Geometry: final body of the model. Coordinates: model frame, mm. A direction names the side the tool comes from. Coordinates: 2 decimals unless noted, no trailing zeros. Order: outer loops, then holes, each group sorted by start corner. A loop starts at its lowest first (then second) coordinate and runs counter-clockwise, first axis right, second up. Notation, with made-up numbers: (-27.75, -34.75) -> (4.25, -34.75) arc R11 ccw to (4.25, -17.75) -> close; hole circle Ø8 at (55.25, -1.75). An arc over 180 degrees is marked (long way). Answer in a Markdown table with one row per item. Add a question column.
1) Section query B-B on y = -0.5. Return the cut outline in (x, z).
2) Section query D-D on z = 15. Return the cut outline in (x, y).
3) Pull-direction query (X, two-part tool) for faces 1 (the face through (-44.113, -3, 18)), 2 (the face through (-31, -3, 44.656)), 3 (the face through (-27.603, -3, 10)); classes: +X half, -X half, draft (parallel to the pull), parting line (faces both ways), or undercut.
4) Contact query for flat-ended pins moving along their axis: P1, Ø3, axis at y = -2.5, z = 36, coming from the +X side; P2, Ø3, axis at x = -32, y = -4, coming from the -Z side; P3, Ø10, axis at x = -31, z = 36, coming from the +Y side; P4, Ø1.9, axis at y = -1.5, z = 18, coming from the -X side. Output: stop coordinate, or through.
5) Section query C-C on x = -26. Return the cut outline in (y, z), then the cut area to 3 significant figures.
6) Set-up query: faces 4 (the face through (-44.113, -3, 34)), 5 (the face through (-28.238, -3, 41)), 6 (the face through (-20, -3, 12.906)), 7 (the face through (-35.223, -3, 10)), 8 (the face through (-50.463, -3, 26)). Return all of +Z, -Z, +X, -X, +Y, -Y with unobstructed straight access to the full face (end or side cutting, diameter ignored); none if empty.
7) Section query A-A on z = 10. Return the cut outline in (x, y).
8) Ray query, line 1 (X direction, y = -4.5, z = 11); line 2 (Z direction, x = -45, y = -1.75); line 3 (Z direction, x = -27, y = -3.5). Return the intervals inside material, ascending. Write a range as from..to.
```python
from build123d import *

# Parameters (mm, degrees)
F0_W     = 6.35
F0_H     = 6.35
F1_DEPTH = 6.35


with BuildPart() as f1:
    # F0 (on Front) → F1 (new body)
    with BuildSketch(Plane.XZ):
        Polygon((-34.587686, 38.306355), (-44.112686, 38.306355), (-44.112686, 28.781355), (-44.112686, 22.431355), (-44.112686, 12.906355), (-41.572686, 12.906355), (-35.222686, 12.906355), (-27.602686, 12.906355), (-21.252686, 12.906355), (-18.712686, 12.906355), (-18.712686, 22.431355), (-18.712686, 28.781355), (-18.712686, 38.306355), (-28.237686, 38.306355), align=None)
        with Locations((-31.412686, 41.481355)):
            Rectangle(F0_W, F0_H)
        with Locations((-47.287686, 25.606355)):
            Rectangle(F0_W, F0_H)
        with Locations((-15.537686, 25.606355)):
            Rectangle(F0_W, F0_H)
        with Locations((-38.397686, 9.731355)):
            Rectangle(F0_W, F0_H)
        with Locations((-24.427686, 9.731355)):
            Rectangle(F0_W, F0_H)
    extrude(amount=F1_DEPTH)


solid = f1.part
```
Result:
| question | item | result |
|---|---|---|
| 1 | outline | (-50.46, 22.43) -> (-44.11, 22.43) -> (-44.11, 12.91) -> (-41.57, 12.91) -> (-41.57, 6.56) -> (-35.22, 6.56) -> (-35.22, 12.91) -> (-27.6, 12.91) -> (-27.6, 6.56) -> (-21.25, 6.56) -> (-21.25, 12.91) -> (-18.71, 12.91) -> (-18.71, 22.43) -> (-12.36, 22.43) -> (-12.36, 28.78) -> (-18.71, 28.78) -> (-18.71, 38.31) -> (-28.24, 38.31) -> (-28.24, 44.66) -> (-34.59, 44.66) -> (-34.59, 38.31) -> (-44.11, 38.31) -> (-44.11, 28.78) -> (-50.46, 28.78) -> close |
| 2 | outline | (-44.11, -6.35) -> (-18.71, -6.35) -> (-18.71, 0) -> (-44.11, 0) -> close |
| 3 | face 1 | -X half |
| 3 | face 2 | draft |
| 3 | face 3 | undercut |
| 4 | P1 | x = -18.71 |
| 4 | P2 | z = 12.91 |
| 4 | P3 | y = 0 |
| 4 | P4 | x = -44.11 |
| 5 | outline | (-6.35, 6.56) -> (0, 6.56) -> (0, 38.31) -> (-6.35, 38.31) -> close |
| 5 | area | 202 mm2 |
| 6 | face 4 | +Z, -X, +Y, -Y |
| 6 | face 5 | +Z, +X, +Y, -Y |
| 6 | face 6 | -Z, +X, +Y, -Y |
| 6 | face 7 | -Z, +Y, -Y |
| 6 | face 8 | +Z, -Z, -X, +Y, -Y |
| 7 | outline | (-41.57, -6.35) -> (-35.22, -6.35) -> (-35.22, 0) -> (-41.57, 0) -> close; (-27.6, -6.35) -> (-21.25, -6.35) -> (-21.25, 0) -> (-27.6, 0) -> close |
| 8 | line 1 | -41.57..-35.22, -27.6..-21.25 |
| 8 | line 2 | 22.43..28.78 |
| 8 | line 3 | 6.56..38.31 |
